Verification items for the finished model (mm, model axes). Face numbers are marked on the shaded views. A direction names the side the tool comes from. Give positions to 0.01 mm unless a question says otherwise; leave off trailing zeros. Loops run counter-clockwise (first coordinate to the right, second up) from the corner with the lowest first, then second, coordinate; pieces in that order, holes last. Notation, with made-up numbers: M -3.5,40 L 41.5,40 A30 cw 41.5,77 Z; hole C -3.5,52 d11. An arc over 180 degrees is marked long. Use a Markdown table: item, result.
Autodesk Inventor part; units mm, degrees
ref_plane "YZ Plane" through (0, 0, 0) normal (1, 0, 0) x (0, 1, 0)
ref_plane "XZ Plane" through (0, 0, 0) normal (0, 1, 0) x (-1, 0, 0)
ref_plane "XY Plane" through (0, 0, 0) normal (0, 0, 1) x (1, 0, 0)
sketch "Sketch1" plane through (0, 0, 0) normal (0, 0, 1) x (1, 0, 0)
  arc A0 (-26.899996, 0.000091) -> (-32.192027, -2.19194) centre (-29.999996, 0.000091) ccw
  arc A1 (32.192013, -2.19194) -> (26.899982, 0.000091) centre (29.999982, 0.000091) ccw
  arc A2 (-25.499996, 0.000091) -> (-33.099996, 3.261992) centre (-29.999996, 0.000091) ccw
  arc A3 (33.181962, -3.181889) -> (34.499982, 0.000091) centre (29.999982, 0.000091) ccw
  line L0 (-29.999996, 0.000091) -> (-35.729952, -5.729865)
  line L1 (-29.999996, 0.000091) -> (-21.896614, 0.000091) construction
  line L2 (29.999982, 0.000091) -> (35.185041, -5.184968)
  line L3 (29.999982, 0.000091) -> (37.332763, 0.000091) construction
  line L4 (-29.999996, 0.000091) -> (29.999982, 0.000091)
  line L5 (-34.499996, 0.000255) -> (-34.499996, 20.000255)
  line L6 (-34.499996, 20.000255) -> (34.499982, 20.000255)
  line L7 (34.499982, 20.000255) -> (34.499982, 0.000091)
  line L8 (-31.099996, 18) -> (31.099982, 18)
  line L9 (33.099982, 16) -> (33.099982, 3.261992)
  arc A4 (-33.099996, 3.261992) -> (-34.499996, 0.000091) centre (-29.999996, 0.000091) ccw
  line L10 (-33.099996, 3.261992) -> (-33.099996, 16)
  arc A5 (33.099982, 3.261992) -> (25.499982, 0.000091) centre (29.999982, 0.000091) ccw
  arc A6 (-34.499996, -0.000073) -> (-33.181977, -3.181889) centre (-29.999996, 0.000091) ccw
  arc A7 (-34.499996, 0.000091) -> (-34.499996, -0.000073) centre (-29.999996, 0.000091) ccw
  arc A8 (-33.099996, 7.640683) -> (-29.95922, 4.499906) centre (-30.103466, 7.496437) ccw
  line L11 (-29.95922, 4.499906) -> (-33.099996, 7.640683) construction
  line L12 (-29.95922, 4.499906) -> (-25.517491, 4.499906) construction
  arc A9 (29.959205, 4.499906) -> (33.099982, 7.640683) centre (30.103452, 7.496437) ccw
  line L13 (29.959205, 4.499906) -> (33.099982, 7.640683) construction
  line L14 (29.959205, 4.499906) -> (34.400934, 4.499906) construction
  arc A10 (-31.099996, 18) -> (-33.099996, 16) centre (-31.099996, 16) ccw
  arc A11 (33.099982, 16) -> (31.099982, 18) centre (31.099982, 16) ccw
  point P0 (0, 0)
  point P1 (-33.099996, 18)
  point P2 (33.099982, 18)
  point P3 (-30.164953, 4.497067)
  point P4 (-33.099996, 7.35219)
  point P5 (33.099982, 7.35219)
  point P6 (30.164938, 4.497067)
  dimension "d0" = 6.2
  dimension "d1" = 6.2
  dimension "d2" = 9
  dimension "d3" = 9
  dimension "d4" = 135
  dimension "d5" = 45
  dimension "d6" = 20
  dimension "d17" = 135
  dimension "d18" = 3
  dimension "d19" = 45
  dimension "d20" = 3
  dimension "d23" = 2
extrude "Extrusion1" add sketch "Sketch1" along normal blind 75 contours A0 L0 A6 A4 A2 A8 L4 | A8 A2 | A5 A9 L9 A11 L8 A10 L10 A4 L5 L6 L7 A3 L2 A1 L4 | A5 A9
fillet "Fillet1" radius 2 2 edges at (-34.5, 20.0003, 37.5) (34.5, 20.0003, 37.5)
sketch "Sketch1 outline for Extrusion3" plane through (0, 0, 0) normal (0, 0, 1) x (1, 0, 0)
  arc A0 (-30.164953, 4.497067) -> (-33.099996, 7.35219) centre (-30.103466, 7.496437) cw
  arc A1 (-33.099996, 3.261992) -> (-30.164953, 4.497067) centre (-29.999996, 0.000091) cw
  line L0 (-33.099996, 7.35219) -> (-33.099996, 3.261992)
  arc A2 (33.099982, 7.35219) -> (30.164938, 4.497067) centre (30.103452, 7.496437) cw
  line L1 (33.099982, 3.261992) -> (33.099982, 7.35219)
  arc A3 (30.164938, 4.497067) -> (33.099982, 3.261992) centre (29.999982, 0.000091) cw
extrude "Extrusion3" add sketch "Sketch1 outline for Extrusion3" along normal blind 75
ref_plane "Work Plane1" through (-33.099996, -4, 0) normal (0, -1, 0) x (1, 0, 0)
sketch "Sketch2" plane through (-33.099996, -4, 0) normal (0, -1, 0) x (1, 0, 0)
  line L0 (73.099996, 5) -> (-6.900004, 5)
  line L1 (-6.900004, 5) -> (-6.900004, 70)
  line L2 (-6.900004, 70) -> (73.099996, 70)
  line L3 (73.099996, 70) -> (73.099996, 5)
  line L4 (73.099996, 5) -> (-6.900004, 70) construction
  line L5 (-6.900004, 5) -> (73.099996, 70) construction
  point P0 (33.099996, 0)
  point P1 (33.099996, 37.5)
  dimension "d12" = 80
  dimension "d13" = 65
  dimension "d14" = 37.5
extrude "Extrusion2" cut sketch "Sketch2" against normal blind 15
sketch "Sketch3" plane through (0, 0, 75) normal (0, 0, 1) x (1, 0, 0)
  line L0 (34.499982, 0.000091) -> (34.499982, 18.000255)
  line L1 (-32.499996, 20.000255) -> (32.499982, 20.000255)
  line L2 (34.499982, 18.000255) -> (34.499982, 3.146922)
  line L3 (34.499982, 3.146922) -> (-34.499996, 3.146922)
  line L4 (-34.499996, 3.146922) -> (-34.499996, 18.000255)
  arc A0 (-32.499996, 20.000255) -> (-34.499996, 18.000255) centre (-32.499996, 18.000255) ccw
  arc A1 (34.499982, 18.000255) -> (32.499982, 20.000255) centre (32.499982, 18.000255) ccw
  point P0 (0, 0)
  dimension "d24" = 2
extrude "Extrusion4" add sketch "Sketch3" against normal blind 2
sketch "Sketch4" plane through (0, 0, 0) normal (0, 0, -1) x (-1, 0, 0)
  line L0 (34.499996, 20.000255) -> (-34.499982, 20.000255)
  line L1 (-34.499982, 20.000255) -> (-34.499982, 0.000091)
  line L2 (34.499996, 0.000255) -> (34.499996, 20.000255)
  line L3 (34.499996, 18.000255) -> (34.499996, 0.000255)
  line L4 (-32.499982, 20.000255) -> (32.499996, 20.000255)
  line L5 (34.499996, 18.000255) -> (34.499996, 3.117372)
  line L6 (34.499996, 3.117372) -> (-34.499982, 3.117372)
  line L7 (-34.499982, 3.117372) -> (-34.499982, 18.000255)
  arc A0 (-32.499982, 20.000255) -> (-34.499982, 18.000255) centre (-32.499982, 18.000255) ccw
  arc A1 (34.499996, 18.000255) -> (32.499996, 20.000255) centre (32.499996, 18.000255) ccw
  point P0 (0, 0)
  point P1 (-34.499982, 3.117372)
  dimension "d27" = 2
extrude "Extrusion5" add sketch "Sketch4" against normal blind 2 contours A1 L2 L6 L1 A0 L0
properties part number "Cage60mm-Boxy"
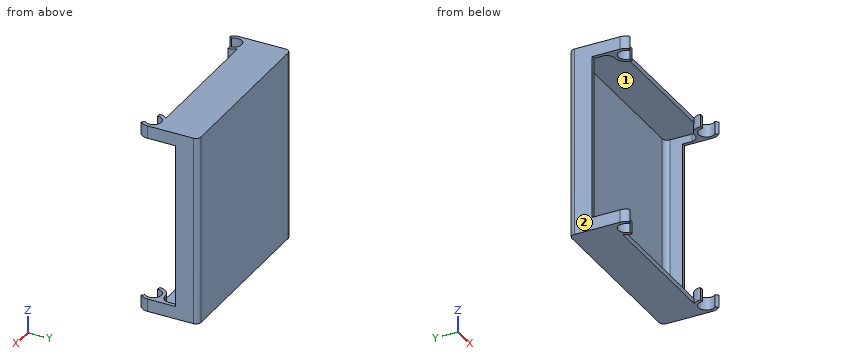
(1) Cross-section at A-A on y = 9.5. Record the cut outline in (x, z).
Results below:
| item | result |
|---|---|
| outline | M -34.5,0 L 34.5,0 L 34.5,5 L 33.1,5 L 33.1,2 L -33.1,2 L -33.1,5 L -34.5,5 Z; M -34.5,70 L -33.1,70 L -33.1,73 L 33.1,73 L 33.1,70 L 34.5,70 L 34.5,75 L -34.5,75 Z |
(2) Cross-section at B-B on x = 15. Record the cut outline in (y, z), then the cut area to 3 significant figures.
Results below:
| item | result |
|---|---|
| outline | M 3.12,0 L 20,0 L 20,75 L 3.15,75 L 3.15,73 L 18,73 L 18,2 L 3.12,2 Z |
| area | 209 mm^2 |
(3) Material ranges on line 1 (X direction, y = 11.25, z = 18.5); line 2 (Z direction, x = 4, y = 8.75); line 3 (Z direction, x = -27.5, y = 3.5), recorded low to high.
Results below:
| item | result |
|---|---|
| line 1 | -34.5 to -33.1, 33.1 to 34.5 |
| line 2 | 0 to 2, 73 to 75 |
| line 3 | 0 to 5, 70 to 75 |
(4) Cross-section at D-D on x = -28. Record the cut outline in (y, z).
Results below:
| item | result |
|---|---|
| outline | M 2.37,0 L 20,0 L 20,75 L 2.37,75 L 2.37,70 L 4.03,70 L 4.03,73 L 18,73 L 18,2 L 4.03,2 L 4.03,5 L 2.37,5 Z |
(5) Set-up check for the marked faces 1 and 2: record each of +Z, -Z, +X, -X, +Y, -Y from which the full face is reachable in a straight line by a thin tool's end or side.
Results below:
| item | result |
|---|---|
| face 1 | none |
| face 2 | +Z, -Z, -X, +Y, -Y |
(6) Cross-section at C-C on z = 34. Record the cut outline in (x, y).
Results below:
| item | result |
|---|---|
| outline | M -34.5,11 L -33.1,11 L -33.1,16 A2 cw -31.1,18 L 31.1,18 A2 cw 33.1,16 L 33.1,11 L 34.5,11 L 34.5,18 A2 ccw 32.5,20 L -32.5,20 A2 ccw -34.5,18 Z |
(7) Gauge pin test, flat ends, axial feed: P1, Ø4.5, axis at x = 31.5, y = 2, coming from the +Z side; P2, Ø5, axis at x = 30, y = 0, coming from the +Z side; P3, Ø1.1, axis at x = -26, z = 73.5, coming from the -Y side; P4, Ø0.7, axis at x = 34, z = 22.5, coming from the -Y side. Record the tip position at first contact, or that the pin passes through.
Results below:
| item | result |
|---|---|
| P1 | z = 75 |
| P2 | through |
| P3 | y = 0 |
| P4 | y = 11 |
